Geometry: see drawing. Coordinates: mm, zero at the bounding-box minimum. A direction names the side the tool comes from. Give positions to 0.01 mm unless a question says otherwise; leave off trailing zeros. Loops run counter-clockwise (first coordinate to the right, second up) from the corner with the lowest first, then second, coordinate; pieces in that order, holes last. Notation, with made-up numbers: M 0,-35.75 L 5,-35.75 A28 ccw 5,-8.75 Z; hole C 49,85.5 d2. An arc over 180 degrees is marked long. Put each result on its own line as item: value.
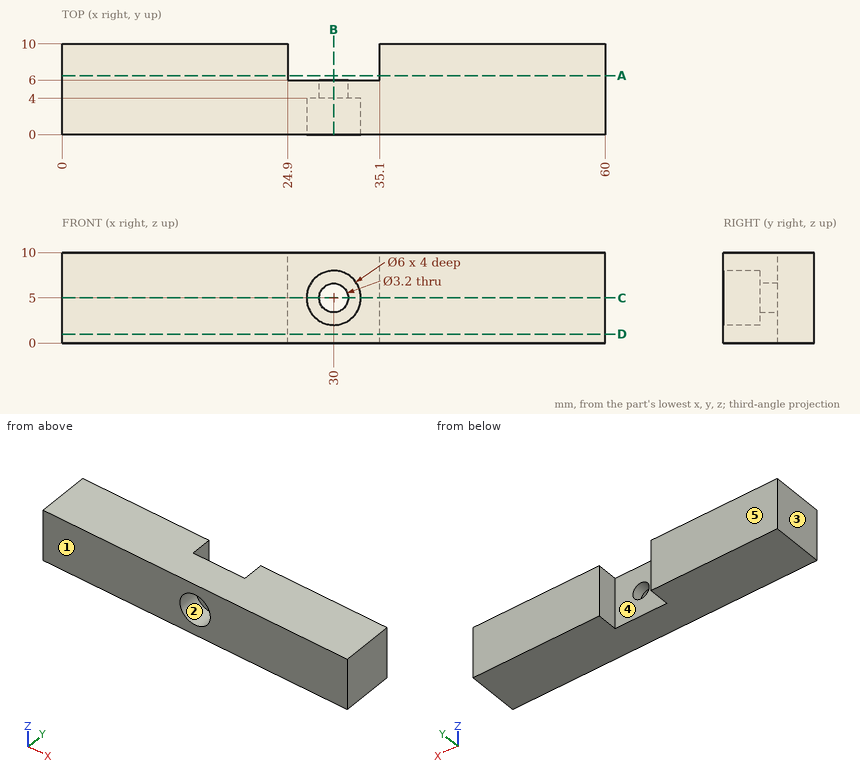
Item 1: Section A-A on y = 6.5. Output: boundary loops of the cut face in (x, z), then the cut area to 3 significant figures.
Output values:
outline: M 0,0 L 24.9,0 L 24.9,10 L 0,10 Z; M 35.1,0 L 60,0 L 60,10 L 35.1,10 Z
area: 498 mm²
Item 2: Section C-C on z = 5. Output: boundary loops of the cut face in (x, y).
Output values:
outline: M 0,0 L 27,0 L 27,4 L 28.4,4 L 28.4,6 L 24.9,6 L 24.9,10 L 0,10 Z; M 31.6,4 L 33,4 L 33,0 L 60,0 L 60,10 L 35.1,10 L 35.1,6 L 31.6,6 Z
Item 3: Pin query (flat end, axial travel): pin 1 Ø3 at (y, z) = (8, 3) entering from -X; pin 2 Ø3.5 at (x, z) = (30, 5) entering from +Y. Return the tip coordinate at first contact, or that it passes through.
Output values:
pin 1: x = 0
pin 2: y = 6
Item 4: Section B-B on x = 30. Output: boundary loops of the cut face in (y, z), then the cut area to 3 significant figures.
Output values:
outline: M 0,0 L 6,0 L 6,3.4 L 4,3.4 L 4,2 L 0,2 Z; M 0,8 L 4,8 L 4,6.6 L 6,6.6 L 6,10 L 0,10 Z
area: 29.6 mm²
Item 5: Mould query, pull axis X, two halves, no side actions, for the marked faces 1, 2 and 3. Classes: pulls with the +X half, pulls with the -X half, needs draft (parallel to the pull), parting line crosses it, or undercut.
Output values:
face 1: needs draft
face 2: undercut
face 3: pulls with the -X half
Item 6: Section D-D on z = 1. Output: boundary loops of the cut face in (x, y).
Output values:
outline: M 0,0 L 60,0 L 60,10 L 35.1,10 L 35.1,6 L 24.9,6 L 24.9,10 L 0,10 Z
Item 7: Set-up query: the marked faces 4 and 5. Return all of +Z, -Z, +X, -X, +Y, -Y with unobstructed straight access to the full face (end or side cutting, diameter ignored); none if empty.
Output values:
face 4: +Z, -Z, +Y
face 5: +Z, -Z, +X, -X, +Y
Item 8: Line query: probe 1 along X at (y, z) = (8, 8.5); probe 2 along X at (y, z) = (5, 5); probe 3 along Y at (x, z) = (29.5, 7.5). Output: solid intervals per line, ascending. Write a range as [from, to].
Output values:
probe 1: [0, 24.9], [35.1, 60]
probe 2: [0, 28.4], [31.6, 60]
probe 3: [4, 6]
